from build123d import *

# Parameters (mm, degrees)
SKETCH1_W           = 10
SKETCH1_H           = 50
BOSS_EXTRUDE1_DEPTH = 30
BOSS_EXTRUDE2_DEPTH = 10
CHAMFER1_SIZE       = 10
CHAMFER2_SIZE       = 15
BOSS_EXTRUDE3_DEPTH = 10


with BuildPart() as part:
    # Sketch1 → Boss-Extrude1 (new body)
    with BuildSketch(Plane(origin=(0, 0, 0), x_dir=(1, 0, 0), z_dir=(0, 1, 0))):
        with Locations((5, 25)):
            Rectangle(SKETCH1_W, SKETCH1_H)
    extrude(amount=BOSS_EXTRUDE1_DEPTH)

    # Sketch1<3> → Boss-Extrude2 (add)
    with BuildSketch(Plane(origin=(0, 0, 0), x_dir=(1, 0, 0), z_dir=(0, 1, 0))):
        Polygon((10, 50), (10, 0), (50, 0), (50, 20), (40, 20), (40, 50), align=None)
    extrude(amount=BOSS_EXTRUDE2_DEPTH)

    # Chamfer1
    chamfer1_edges = [part.edges().sort_by_distance(p)[0] for p in [
        (50, 5, 0),
    ]]
    chamfer(chamfer1_edges, length=CHAMFER1_SIZE)

    # Chamfer2
    chamfer2_edges = [part.edges().sort_by_distance(p)[0] for p in [
        (5, 30, -50),
    ]]
    chamfer(chamfer2_edges, length=CHAMFER2_SIZE)

    # Sketch2 → Boss-Extrude3 (add)
    with BuildSketch(Plane.XY):
        Polygon((10, 10), (30, 10), (10, 30), align=None)
    extrude(amount=-BOSS_EXTRUDE3_DEPTH)


solid = part.part
Here's how the part is built. I have some questions about the finished solid (model axes, mm). A direction names the side the tool comes from. Coordinates: 2 decimals unless noted, no trailing zeros. Write each loop counter-clockwise with the first axis right and the second up, starting at its lowest first coordinate (ties: lowest second). Pieces come first, ordered by that corner, then holes.
Item 1: On a 3-axis mill with a long thin cutter (end or side, diameter ignored), from which of +Z, -Z, +X, -X, +Y, -Y can I reach the whole of each face in a straight line? I mean faces 1 (the flat face through (5, 22, -43)), 2 (the flat face through (30, 10, -25)), 3 (the flat face through (40, 5, -35)). Say none if no direction works.
Item 2: Will these pins go through, and if not, where does the flat tip stop? pin 1 (6 mm diameter, centred on x = 35, z = -24, fed in from +Y); pin 2 (8 mm diameter, centred on x = 47.5, y = 6, fed in from -Z); pin 3 (10 mm diameter, centred on x = 22.5, y = 15.5, fed in from -Z); pin 4 (3 mm diameter, centred on x = 34.5, y = 12.5, fed in from +Z).
Item 3: I want a section at B-B on x = 25.5. Write out the boundary of the cut face in (y, z), and give its area (3 significant figures).
Item 4: I want a section at C-C on x = 35.5. Write out the boundary of the cut face in (y, z).
Item 5: I want a section at D-D on x = 47. Write out the boundary of the cut face in (y, z), and give its area (3 significant figures).
Item 6: I want a section at A-A on z = -4.5. Write out the boundary of the cut face in (x, y), and give its area (3 significant figures).
Item 7: If I drill on line 1 (Y direction, x = 39.5, z = -15); line 2 (X direction, y = 4, z = -41); line 3 (Z direction, x = 19, y = 19), over which ranges is the centre line in solid material (lowest first)?
Findings below:
1. face 1: -Z, +X, -X, +Y
1. face 2: -Z, +X, +Y
1. face 3: -Z, +X, +Y, -Y
2. pin 1: stops at y = 10
2. pin 2: stops at z = -20
2. pin 3: stops at z = -10
2. pin 4: passes through
3. outline: (0, -50) - (10, -50) - (10, -10) - (14.5, -10) - (14.5, 0) - (0, 0) - close
3. area: 545 mm2
4. outline: (0, -50) - (10, -50) - (10, 0) - (0, 0) - close
5. outline: (0, -20) - (10, -20) - (10, -7) - (0, -7) - close
5. area: 130 mm2
6. outline: (0, 0) - (44.5, 0) - (44.5, 10) - (30, 10) - (10, 30) - (0, 30) - close
6. area: 845 mm2
7. line 1: y = 0 to 10
7. line 2: x = 0 to 40
7. line 3: z = -10 to 0
